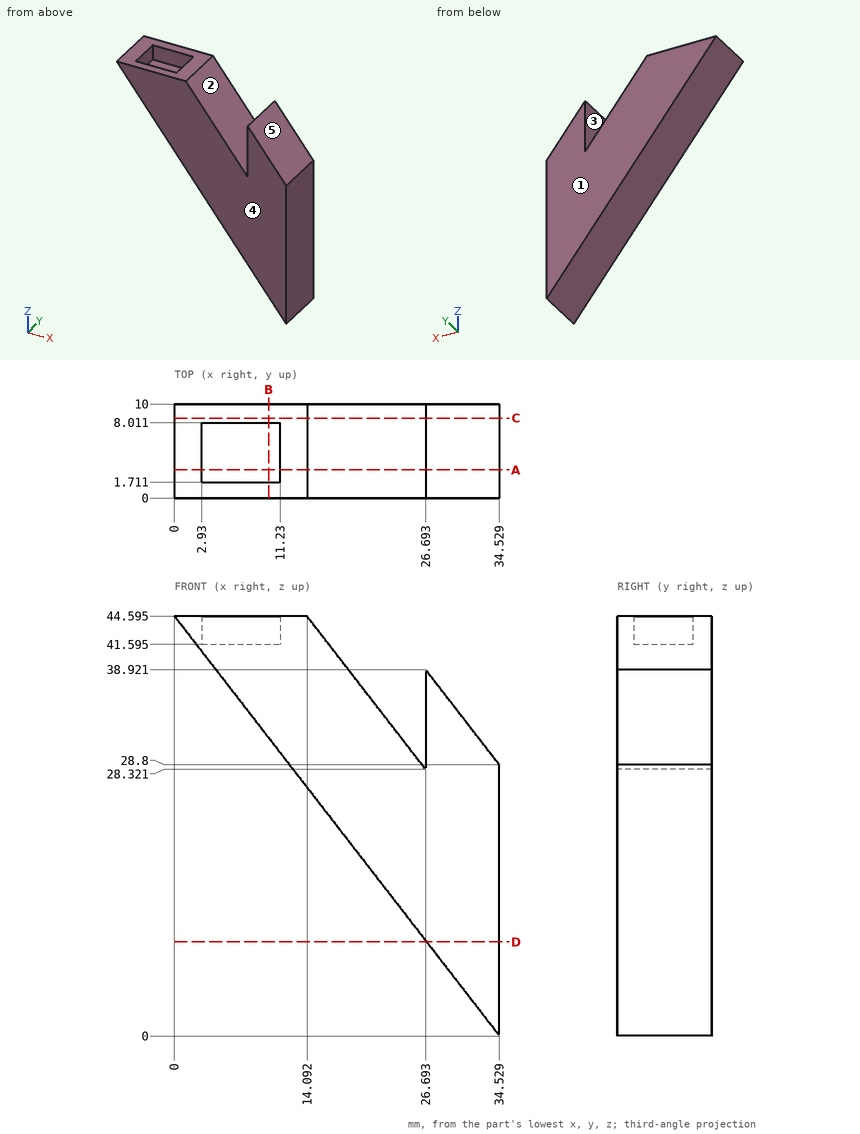
Input: dimensioned drawing with shaded views. Units: mm. Origin: part minimum x, y, z. A direction names the side the tool comes from. Give positions to 0.01 mm unless a question says otherwise; leave off trailing zeros. Write each loop counter-clockwise with the first axis right and the second up, starting at its lowest first coordinate (ties: lowest second). Pieces come first, ordered by that corner, then holes. Notation, with made-up numbers: M 53.25,40 L 93.25,40 A27 cw 93.25,63 Z; hole C 73,-11 d8. An arc over 180 degrees is marked long. Write item = value, one per line. Start each with the question number.
1) First-contact query: pin 1 Ø1.5 at (x, y) = (23.5, 8.5) entering from -Z (1 decimal); pin 2 Ø1.5 at (x, y) = (30.5, 6) entering from +Z; pin 3 Ø5 at (y, z) = (3, 36) entering from -X. Flat tips, straight axial feed; report the tip coordinate or a pass-through.
2) Cut plane D-D on z = 10. Return the cut outline in (x, y).
3) Cut plane A-A on y = 3. Return the cut outline in (x, z) (1 decimal).
4) Cut plane C-C on y = 8.5. Return the cut outline in (x, z) (1 decimal).
5) Draft query along X for the marked faces 3, 4 and 5. Return one class per face: +X half, -X half, draft (parallel to the pull), parting line (faces both ways), or undercut.
6) Cut plane B-B on x = 10. Return the cut outline in (y, z) (1 decimal).
7) Material intervals for line 1 along Y through (x, z) = (9, 42); line 2 along X through (y, z) = (2.5, 30); line 3 along X through (y, z) = (2, 34) (1 decimal), sorted ascending. Write a range as [from, to].
8) Reachability of the marked faces 1 and 2 from +Z, -Z, +X, -X, +Y, -Y: full face, straight path, thin tool, end or side. Return the list, or none.
Solved:
q1.pin_1 = 13.3
q1.pin_2 = 34.97
q1.pin_3 = 4.72
q2.outline = M 26.79,0 L 34.53,0 L 34.53,10 L 26.79,10 Z
q3.outline = M 0,44.6 L 34.5,0 L 34.5,28.8 L 26.7,38.9 L 26.7,28.3 L 14.1,44.6 L 11.2,44.6 L 11.2,41.6 L 2.9,41.6 L 2.9,44.6 Z
q4.outline = M 0,44.6 L 34.5,0 L 34.5,28.8 L 26.7,38.9 L 26.7,28.3 L 14.1,44.6 Z
q5.face_3 = undercut
q5.face_4 = draft
q5.face_5 = +X half
q6.outline = M 0,31.7 L 10,31.7 L 10,44.6 L 8,44.6 L 8,41.6 L 1.7,41.6 L 1.7,44.6 L 0,44.6 Z
q7.line_1 = [0, 1.71], [8.01, 10]
q7.line_2 = [11.3, 25.39], [26.69, 33.6]
q7.line_3 = [8.2, 22.3], [26.7, 30.5]
q8.face_1 = +Z, -Z, +X, -X, +Y
q8.face_2 = +Z, +Y, -Y
